```python
from build123d import *

# Parameters (mm, degrees)
F0_R      = 5.5
F1_DEPTH  = 12
F2_R      = 1
F3_R      = 1.98573
F4_DEPTH  = 5
F6_R      = 6.124075
F7_DEPTH  = 6
F8_R      = 5.5
F7_FACE_R = 0.624075
F9_DEPTH  = 4
F10_R     = 2.813171
F11_DEPTH = 18
F12_SIZE  = 1


with BuildPart() as f1:
    # F0 (on Top) → F1 (new body)
    with BuildSketch(Plane.XY):
        Circle(F0_R)
    extrude(amount=F1_DEPTH)

    # F2
    f2_edges = [f1.edges().sort_by_distance(p)[0] for p in [
        (-5.5, 0, 12),
    ]]
    fillet(f2_edges, radius=F2_R)

    # F3 (on face) → F4 (join)
    with BuildSketch(Plane(origin=(0, 0, 0), x_dir=(1, 0, 0), z_dir=(0, 0, -1))):
        Circle(F3_R)
    extrude(amount=F4_DEPTH)

    # F6 (on offset) → F7 (join)
    with BuildSketch(Plane.XY.offset(-2.5)):
        Circle(F6_R)
    extrude(amount=-F7_DEPTH)

    # F8
    f8_edges = [f1.edges().sort_by_distance(p)[0] for p in [
        (-6.124075, 0, -8.5),
    ]]
    fillet(f8_edges, radius=F8_R)

    # F7_face (on face) → F9 (cut)
    with BuildSketch(Plane(origin=(0, 0, -8.5), x_dir=(1, 0, 0), z_dir=(0, 0, -1))):
        Circle(F7_FACE_R)
    extrude(amount=-F9_DEPTH, mode=Mode.SUBTRACT)

    # F10 (on Right) → F11 (join)
    with BuildSketch(Plane.YZ):
        with Locations((0, 6.498161)):
            Circle(F10_R)
    extrude(amount=F11_DEPTH)

    # F12
    f12_edges = [f1.edges().sort_by_distance(p)[0] for p in [
        (18, -2.813171, 6.498161),
    ]]
    chamfer(f12_edges, length=F12_SIZE)


solid = f1.part
```
Could you check a few things on this model? Use its own coordinates, in mm. A direction names the side the tool comes from. Round coordinates to 2 decimals unless told otherwise and drop trailing zeros. Loops run counter-clockwise (first coordinate to the right, second up) from the corner with the lowest first, then second, coordinate; pieces in that order, holes last. Notation, with made-up numbers: (59, -3.75) - (102, -3.75) arc R24 cw to (102, 11.25) - close; hole circle Ø8 at (-20.5, -14). An arc over 180 degrees is marked (long way). Answer in a Markdown table with one row per item. Add a question column.
(1) If we mould it in two halves opening along X, with no side actions, what happens to faces 1 (the face through (0, 0, -4.5)), 2 (the face through (0.595, -0.187, -6.528)), 3 (the face through (-1.576, 1.208, -1.232)), 4 (the face through (0, 0, 12))? For each: pulls with the +X half, pulls with the -X half, needs draft (parallel to the pull), parting line crosses it, or undercut.
(2) If we section it at A-A (z = 3): Please give me the cut outline in (x, y), plus the area to 3 significant figures.
(3) For faces 5 (the face through (10.777, -0.366, 9.287)), 6 (the face through (0, -3, -2.5)), 7 (the face through (5.84, 1.84, -2.75)), which set-ups out of +Z, -Z, +X, -X, +Y, -Y let a thin tool reach every point of the face, with its end or its side?
(4) I'm going to push flat-ended pins straight in: pin 1 (1 mm diameter, centred on x = 3, y = -2, fed in from -Z); pin 2 (4 mm diameter, centred on x = 4.5, z = 2.5, fed in from -Y); pin 3 (1.1 mm diameter, centred on x = 0, y = 0, fed in from -Z). Where does each tip first touch, or does it pass through?
(5) If we section it at B-B (x = 9.25): Please give me the cut outline in (y, z).
(6) I need wall thicknesses on line 1 along Y through (x, z) = (0, -5.8); line 2 along Z through (x, y) = (-2, 2.5); line 3 along Z through (x, y) = (-2, 4.5). Which ranges of each line are inside material? Lowest first, please.
Model answer:
| question | item | result |
|---|---|---|
| 1 | face 1 | undercut |
| 1 | face 2 | undercut |
| 1 | face 3 | parting line crosses it |
| 1 | face 4 | needs draft |
| 2 | outline | circle Ø11 at (0, 0) |
| 2 | area | 95.0 mm² |
| 3 | face 5 | +X |
| 3 | face 6 | none |
| 3 | face 7 | -Z |
| 4 | pin 1 | stops at z = -7.91 |
| 4 | pin 2 | stops at y = -4.9 |
| 4 | pin 3 | stops at z = -4.5 |
| 5 | outline | circle Ø5.63 at (0, 6.5) |
| 6 | line 1 | y = -5.36 to -0.62, 0.62 to 5.36 |
| 6 | line 2 | z = -7.86 to -2.5, 0 to 12 |
| 6 | line 3 | z = -6.43 to -2.5, 0 to 11.91 |
